Autodesk Inventor part; units mm, degrees
ref_plane "Start Plane" through (0, 0, 25.4165) normal (0, 0, 1) x (1, 0, 0)
ref_plane "End Plane" through (0, 0, 680.4425) normal (0, 0, 1) x (1, 0, 0)
ref_plane "Work Plane4" through (0, 12.7, 680.4425) normal (0.2991, 0, 0.9542) x (0.9542, 0, -0.2991)
ref_plane "Start Plane" through (0, 0, 25.4165) normal (0, 0, 1) x (1, 0, 0)
ref_plane "End Plane" through (0, 0, 680.4425) normal (0, 0, 1) x (1, 0, 0)
sketch "Sketch" plane through (0, 0, 0) normal (0, 0, 1) x (1, 0, 0)
  line L0 (25.4, 0) -> (0, 0)
  line L1 (0, 0) -> (0, 25.4)
  line L2 (0, 25.4) -> (1.651, 25.4)
  line L3 (3.175, 23.876) -> (3.175, 6.477)
  line L4 (6.477, 3.175) -> (23.876, 3.175)
  line L5 (25.4, 1.651) -> (25.4, 0)
  line L6 (0, -11.0414) -> (0, 31.5385) construction
  line L7 (-11.0414, 0) -> (31.5385, 0) construction
  arc A0 (3.175, 6.477) -> (6.477, 3.175) centre (6.477, 6.477) ccw
  arc A1 (3.175, 23.876) -> (1.651, 25.4) centre (1.651, 23.876) ccw
  arc A2 (25.4, 1.651) -> (23.876, 3.175) centre (23.876, 1.651) ccw
  line L8 (0, 40.0545) -> (0, -19.5574) construction
  line L9 (-19.5574, 0) -> (40.0545, 0) construction
  point P0 (3.175, 25.4)
  point P1 (3.175, 3.175)
  point P2 (25.4, 3.175)
  dimension "d0" = 25.4
  dimension "d1" = 25.4
  dimension "d2" = 3.175
  dimension "d3" = 3.175
  dimension "d10" = 0
  dimension "d11" = 0
  dimension "d14" = 3.302
  dimension "d15" = 1.524
extrude "Body" add sketch "Sketch" along normal up to surface (655.026 mm away) from surface at 25.4165
sketch "Sketch3" plane through (0, 0, 0) normal (0, 0, 1) x (1, 0, 0)
  line L0 (0, 0) -> (10, 0)
ref_plane "Work Plane3" through (0, 0, 0) normal (0, -1, 0) x (1, 0, 0)
ref_plane "Work Plane4" through (0, 12.7, 680.4425) normal (0.2991, 0, 0.9542) x (0.9542, 0, -0.2991)
split "Split1" plane through (0, 12.7, 680.4425) removes the side toward (0.2991, 0, 0.9542)
ref_plane "Work Plane5" through (-0.8564, 664.6, 23.7336) normal (0, 1, 0) x (1, 0, 0)
split "Split2" plane through (-0.8564, 664.6, 23.7336) removes the side toward (0, 1, 0)
sketch "Sketch4" plane through (0, 0, 0) normal (0, -1, 0) x (1, 0, 0)
  line L0 (-2, 25.4165) -> (12, 25.4165)
  line L1 (-2, 680.4425) -> (12, 680.4425)
  dimension "d17" = 655.026
equation "\"d0\" = G_H"
equation "\"d1\" = G_H"
equation "\"d2\" = G_T"
equation "\"d3\" = G_T"
equation "\"d14\" = G_IR"
equation "\"d15\" = G_ER"
equation "\"d4\" = G_L"
equation "\"G_H\" = 25.4"
equation "\"G_T\" = 3.175"
equation "\"G_ER\" = 1.524"
equation "\"G_IR\" = 3.302"
equation "\"G_L\" = d17"
equation "\"ex\" = 0"
equation "\"G_OFFSET_START\" = -25.41653"
equation "\"G_OFFSET_END\" = 0"
equation "\"d12\" = -G_OFFSET_START"
equation "\"d13\" = G_OFFSET_END + B_L"
equation "\"B_L\" = 680.44252"
properties part number "AISC - L 1 x 1 x 1/8 - 25.788" material "Steel, Mild"
Check sheet for the modelled part. Datum: model origin and axes. Units: mm. A direction names the side the tool comes from. Give positions to 0.01 mm unless a question says otherwise; leave off trailing zeros. Write each loop counter-clockwise with the first axis right and the second up, starting at its lowest first coordinate (ties: lowest second). Pieces come first, ordered by that corner, then holes.
Item 1: Gauge pin test, flat ends, axial feed: pin 1 (12 mm diameter, centred on x = 16.5, z = 158.5, fed in from +Y) (3 decimals); pin 2 (4 mm diameter, centred on x = 4, y = 6, fed in from +Z). Record the tip position at first contact, or that the pin passes through.
Item 2: Scan lines: L1, parallel to X at y = 12, z = 117 (3 decimals); L2, parallel to Y at x = 6, z = 239; L3, parallel to Z at x = 1.5, y = 6.5. Record each from-to range of solid material in increasing order.
Item 3: Cross-section at A-A (z = 300). Enter the section's corners in (x, y) (3 decimals), and give its area (3 significant figures).
Item 4: Cross-section at C-C (x = 15.5). Enter the section's corners in (y, z) (1 decimal), and give its area (3 significant figures).
Item 5: Access from +Z, -Z, +X, -X, +Y, -Y to the whole of each face (thin tool, end or side, straight path). Record for faces 1 (the face through (3.175, 15, 348)), 2 (the face through (3, 5, 25.416)).
Item 6: Cross-section at B-B (y = 13.75). Enter the section's corners in (x, z) (1 decimal).
Report:
1. pin 1: stops at y = 3.175
1. pin 2: stops at z = 679.82
2. L1: x = 0 to 3.175
2. L2: y = 0 to 3.21
2. L3: z = 25.42 to 679.97
3. outline: (0, 0) - (25.4, 0) - (25.4, 1.651) arc R1.524 ccw to (23.876, 3.175) - (6.477, 3.175) arc R3.302 cw to (3.175, 6.477) - (3.175, 23.876) arc R1.524 ccw to (1.651, 25.4) - (0, 25.4) - close
3. area: 153 mm2
4. outline: (0, 25.4) - (3.2, 25.4) - (3.2, 675.6) - (0, 675.6) - close
4. area: 2,060 mm2
5. face 1: +Z, -Z, +X, +Y
5. face 2: -Z, +X, -X, +Y, -Y
6. outline: (0, 25.4) - (3.2, 25.4) - (3.2, 679.4) - (0, 680.4) - close
